Can you work these out from the drawing? Everything is in mm from the part's minimum corner. A direction names the side the tool comes from. Give positions to 0.01 mm unless a question says otherwise; leave off trailing zeros. Loops run counter-clockwise (first coordinate to the right, second up) from the corner with the lowest first, then second, coordinate; pieces in that order, holes last.
Q1. If we section it at C-C (y = 14.5): Please give me the cut outline in (x, z), plus the area to 3 significant figures.
Q2. For the marked faces 4, 5 and 6, which set-ups out of +Z, -Z, +X, -X, +Y, -Y let a thin tool reach every point of the face, with its end or its side?
Q3. If we section it at A-A (x = 61): Please give me the cut outline in (y, z).
Q4. If we section it at D-D (y = 38.5): Please give me the cut outline in (x, z), plus the area to 3 significant figures.
Q5. Will these pins go through, and if not, where does the flat tip stop? P1, Ø5, axis at y = 2, z = 338.5, coming from the -X side; P2, Ø12.5, axis at y = 18.5, z = 172, coming from the +X side; P3, Ø3, axis at y = 2, z = 123, coming from the +X side.
Q6. We'd pull the mould along X, two halves only. Please class the marked faces 1, 2 and 3: +X half, -X half, draft (parallel to the pull), parting line (faces both ways), or undercut.
Q7. If we section it at B-B (z = 396.5): Please give me the cut outline in (x, y).
Q8. I need wall thicknesses on line 1 (X direction, y = 26, z = 415); line 2 (Z direction, x = 167.5, y = 36); line 3 (X direction, y = 39, z = 258). Which ranges of each line are inside material? Lowest first, please.
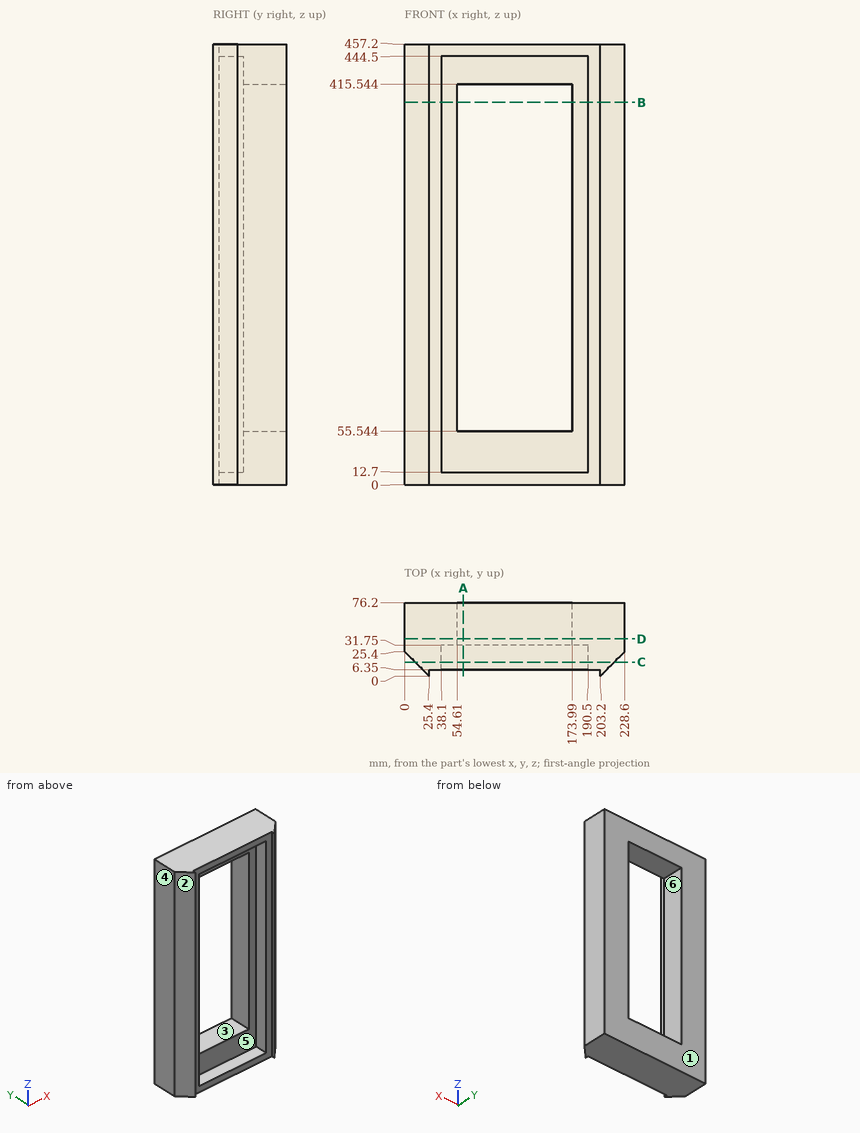
Check sheet entries:
1. outline: (10.9, 0) - (217.7, 0) - (217.7, 457.2) - (10.9, 457.2) - close; hole (38.1, 12.7) - (190.5, 12.7) - (190.5, 444.5) - (38.1, 444.5) - close
1. area: 28,700 mm2
2. face 4: +Z, -Z, -X, +Y, -Y
2. face 5: -Y
2. face 6: +Y, -Y
3. outline: (6.35, 0) - (76.2, 0) - (76.2, 55.54) - (31.75, 55.54) - (31.75, 12.7) - (6.35, 12.7) - close; (6.35, 444.5) - (31.75, 444.5) - (31.75, 415.54) - (76.2, 415.54) - (76.2, 457.2) - (6.35, 457.2) - close
4. outline: (0, 0) - (228.6, 0) - (228.6, 457.2) - (0, 457.2) - close; hole (54.61, 55.54) - (173.99, 55.54) - (173.99, 415.54) - (54.61, 415.54) - close
4. area: 61,500 mm2
5. P1: stops at x = 20.9
5. P2: stops at x = 227.95
5. P3: stops at x = 206.7
6. face 1: draft
6. face 2: -X half
6. face 3: undercut
7. outline: (0, 25.4) - (25.4, 0) - (25.4, 6.35) - (38.1, 6.35) - (38.1, 31.75) - (54.61, 31.75) - (54.61, 76.2) - (0, 76.2) - close; (173.99, 31.75) - (190.5, 31.75) - (190.5, 6.35) - (203.2, 6.35) - (203.2, 0) - (228.6, 25.4) - (228.6, 76.2) - (173.99, 76.2) - close
8. line 1: x = 0 to 38.1, 190.5 to 228.6
8. line 2: z = 0 to 55.54, 415.54 to 457.2
8. line 3: x = 0 to 54.61, 173.99 to 228.6
